Input: dimensioned drawing with shaded views. Units: mm. Origin: part minimum x, y, z. A direction names the side the tool comes from. Coordinates: 2 decimals unless noted, no trailing zeros. Order: outer loops, then holes, each group sorted by start corner. A loop starts at its lowest first (then second) coordinate and runs counter-clockwise, first axis right, second up. Notation, with made-up numbers: (68, -21.5) -> (117, -21.5) arc R14 ccw to (117, 3.5) -> close; hole circle Ø4 at (-7.5, 38). An arc over 180 degrees is marked (long way). Answer in a Markdown table with one row per item. Add a question column.
1) Contact query for flat-ended pins moving along their axis: P1, Ø5, axis at y = 13.25, z = 37.16, coming from the +X side; P2, Ø4, axis at x = 19.5, y = 19, coming from the -Z side (1 decimal); P3, Ø22, axis at y = 30.5, z = 24, coming from the -X side; P4, Ø8.5, axis at y = 39.5, z = 22, coming from the +X side. Output: stop coordinate, or through.
2) Section query D-D on x = 4. Return the cut outline in (y, z).
3) Section query C-C on y = 39.5. Return the cut outline in (x, z).
4) Ray query, line 1 (X direction, y = 20, z = 28.5); line 2 (Z direction, x = 20, y = 22); line 3 (X direction, y = 18, z = 36). Return the intervals inside material, ascending. Write a range as from..to.
5) Section query A-A on z = 22. Return the cut outline in (x, y).
6) Section query B-B on y = 13.25. Return the cut outline in (x, z) (1 decimal).
7) Set-up query: the marked faces 1, 2 and 3. Return all of +Z, -Z, +X, -X, +Y, -Y with unobstructed straight access to the full face (end or side cutting, diameter ignored); none if empty.
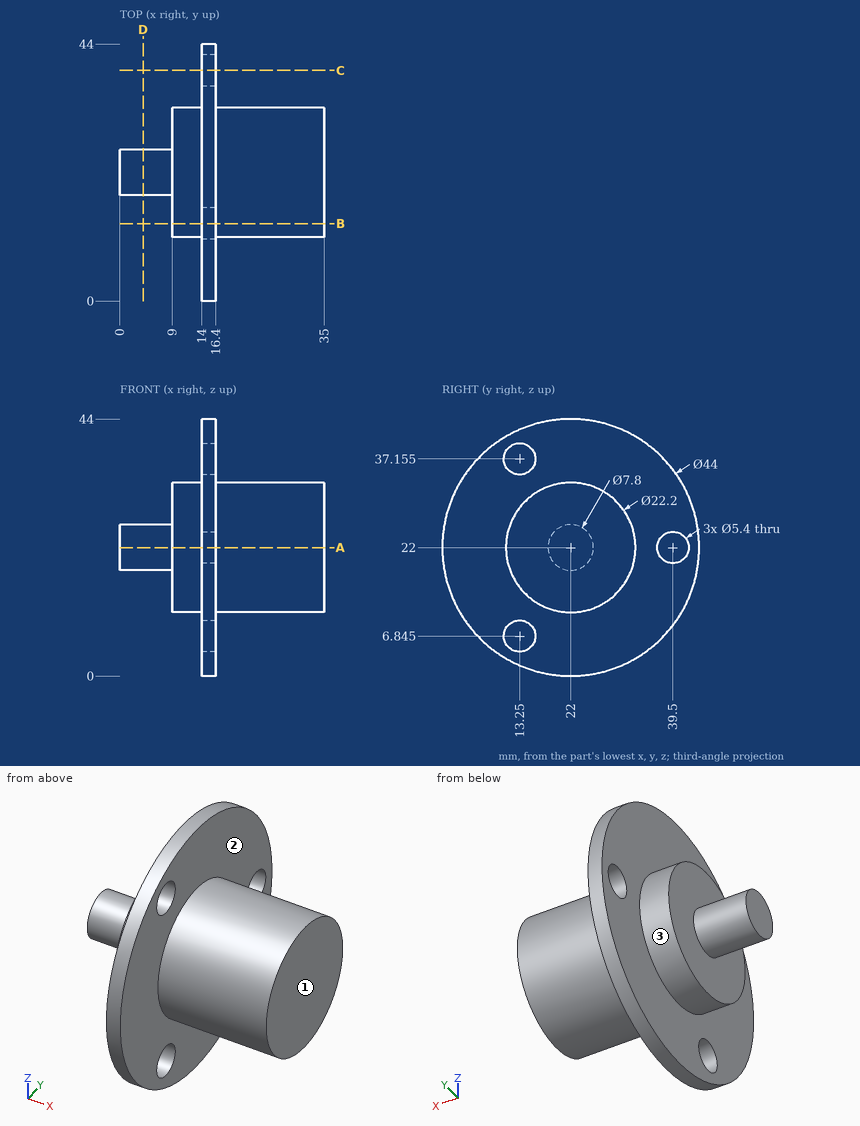
Result:
| question | item | result |
|---|---|---|
| 1 | P1 | through |
| 1 | P2 | z = 10.9 |
| 1 | P3 | x = 0 |
| 1 | P4 | x = 16.4 |
| 2 | outline | circle Ø7.8 at (22, 22) |
| 3 | outline | (14, 8.67) -> (16.4, 8.67) -> (16.4, 19.3) -> (14, 19.3) -> close; (14, 24.7) -> (16.4, 24.7) -> (16.4, 35.33) -> (14, 35.33) -> close |
| 4 | line 1 | 9..35 |
| 4 | line 2 | 10.9..33.1 |
| 4 | line 3 | 14..16.4 |
| 5 | outline | (0, 18.1) -> (9, 18.1) -> (9, 10.9) -> (14, 10.9) -> (14, 0) -> (16.4, 0) -> (16.4, 10.9) -> (35, 10.9) -> (35, 33.1) -> (16.4, 33.1) -> (16.4, 36.8) -> (14, 36.8) -> (14, 33.1) -> (9, 33.1) -> (9, 25.9) -> (0, 25.9) -> close; (14, 42.2) -> (16.4, 42.2) -> (16.4, 44) -> (14, 44) -> close |
| 6 | outline | (9, 15.2) -> (14, 15.2) -> (14, 9.5) -> (16.4, 9.5) -> (16.4, 15.2) -> (35, 15.2) -> (35, 28.8) -> (16.4, 28.8) -> (16.4, 34.5) -> (14, 34.5) -> (14, 28.8) -> (9, 28.8) -> close; (14, 1.8) -> (16.4, 1.8) -> (16.4, 4.1) -> (14, 4.1) -> close; (14, 39.9) -> (16.4, 39.9) -> (16.4, 42.2) -> (14, 42.2) -> close |
| 7 | face 1 | +Z, -Z, +X, +Y, -Y |
| 7 | face 2 | +X |
| 7 | face 3 | -X |
